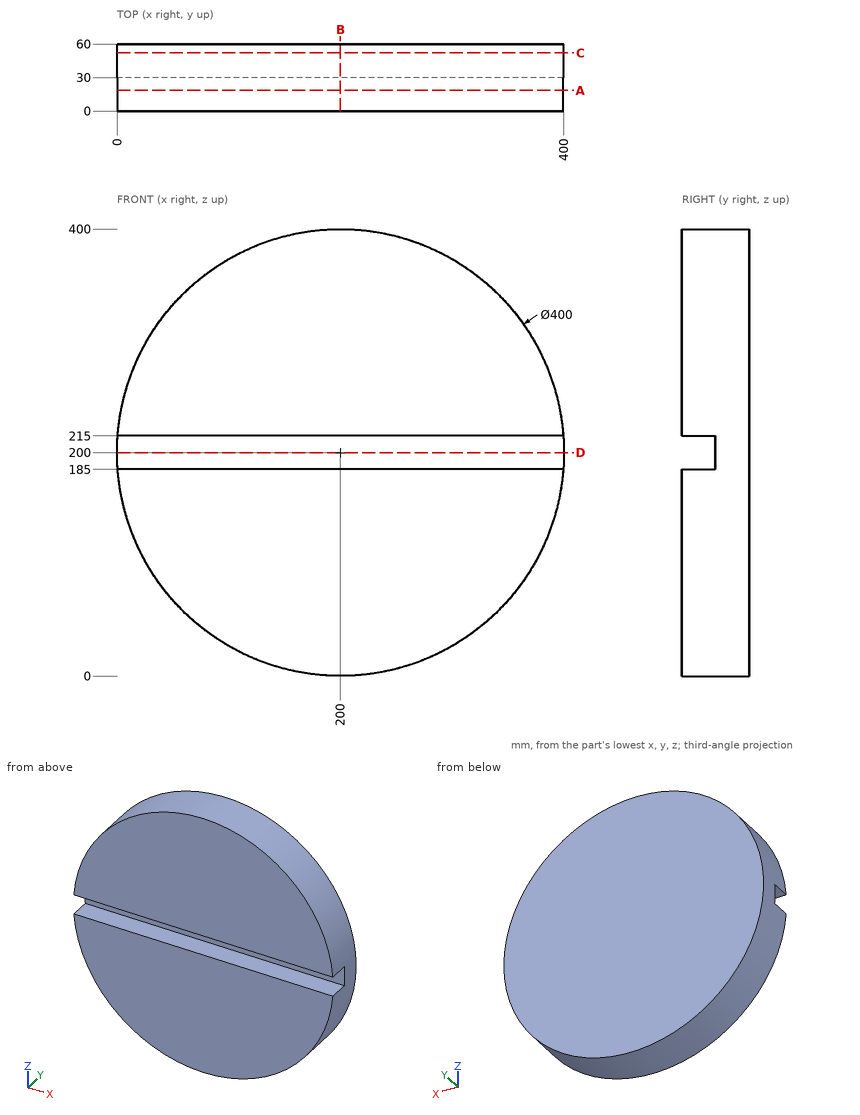
Verification items for this drawing (mm, ordinates from the low corner). Coordinates: 2 decimals unless noted, no trailing zeros. Order: outer loops, then holes, each group sorted by start corner. A loop starts at its lowest first (then second) coordinate and runs counter-clockwise, first axis right, second up. Notation, with made-up numbers: M 48,-25 L 80,-25 A18 ccw 80,-19 Z; hole C 4,66.5 d6. An arc over 180 degrees is marked long. One line per item, written item: value. Start each with the question number.
Item 1: Thickness scan on probe 1 along Z at (x, y) = (283, 7.5); probe 2 along Z at (x, y) = (272.5, 17); probe 3 along X at (y, z) = (48.5, 36.5). Record the ranges inside material, lowest first.
Item 2: Sectioned sample at A-A on y = 18.5. Record the cut outline in (x, z).
Item 3: Sectioned sample at B-B on x = 200. Record the cut outline in (y, z).
Item 4: Sectioned sample at D-D on z = 200. Record the cut outline in (x, y).
Item 5: Depth check by flat-ended pin: P1, Ø1, axis at x = 147.5, y = 13.5, coming from the +Z side; P2, Ø10, axis at x = 60.5, z = 54, coming from the -Y side; P3, Ø3, axis at y = 52, z = 298, coming from the -X side; P4, Ø10, axis at x = 269.5, y = 14, coming from the -Z side. Enter the tip coordinate at first touch or a pass-through.
Item 6: Sectioned sample at C-C on y = 52. Record the cut outline in (x, z), then the cut area to 3 significant figures.
Calculated:
1. probe 1: 18.04 to 185, 215 to 381.96
1. probe 2: 13.6 to 185, 215 to 386.4
1. probe 3: 84.81 to 315.19
2. outline: M 0.56,185 A200 ccw 399.44,185 Z; M 0.56,215 L 399.44,215 A200 ccw Z
3. outline: M 0,0 L 60,0 L 60,400 L 0,400 L 0,215 L 30,215 L 30,185 L 0,185 Z
4. outline: M 0,30 L 400,30 L 400,60 L 0,60 Z
5. P1: z = 393.12
5. P2: y = 0
5. P3: x = 24.82
5. P4: z = 10.69
6. outline: C 200,200 d400
6. area: 126,000 mm^2
